For this review, use the dimensioned drawing (mm, ordinates from the lowest corner) and the shaded views. Coordinates: 2 decimals unless noted, no trailing zeros. Write each loop counter-clockwise with the first axis right and the second up, starting at its lowest first coordinate (ties: lowest second). Pieces come first, ordered by that corner, then holes. Notation, with made-up numbers: (42.5, 29.5) -> (57.5, 29.5) arc R20 cw to (57.5, 49.5) -> close; hole circle Ø9 at (9.5, 80). An arc over 180 degrees is marked (long way). Put each result on its own line as item: value. Start each with the question number.
Item 1: To check wall thickness, follow L1, parallel to Y at x = 68.5, z = 4; L2, parallel to X at y = 7, z = 1.1; L3, parallel to Y at x = 55, z = 0.9. State the ranges of each line that lie inside material, in increasing order.
Item 2: Consider section D-D on x = 30.5. Give the boundary of the cut face in (y, z).
Item 3: Consider section B-B on z = 3.05. Give the boundary of the cut face in (x, y).
Item 4: Consider section C-C on y = 29.5. Give the boundary of the cut face in (x, z), and give its area (3 significant figures).
Item 5: Consider section A-A on y = 8.5. Give the boundary of the cut face in (x, z), and give its area (3 significant figures).
Item 6: Insertion check: P1, Ø1, axis at x = 55, z = 2, coming from the +Y side; P2, Ø1.4, axis at y = 32, z = 2, coming from the -X side; P3, Ø1.4, axis at y = 2, z = 2.5, coming from the -X side. Each pin has a flat end and moves straight along its axis. Give the tip position at first contact, or say it passes through.
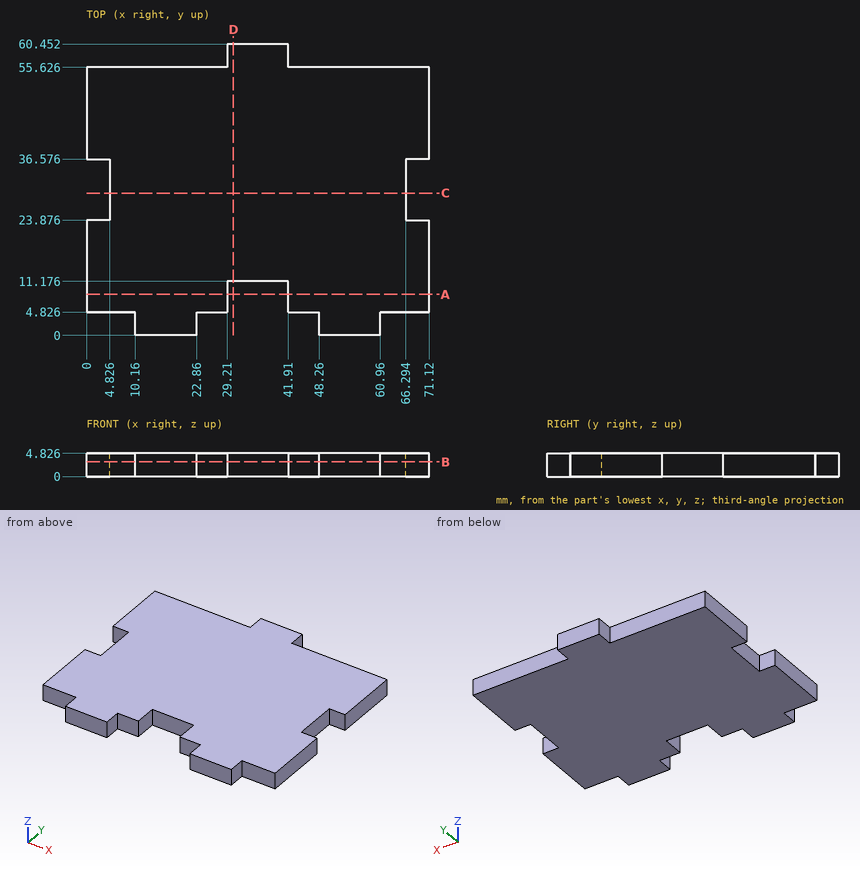
Return value:
1. L1: 4.83 to 23.88, 36.58 to 55.63
1. L2: 0 to 29.21, 41.91 to 71.12
1. L3: 0 to 55.63
2. outline: (11.18, 0) -> (60.45, 0) -> (60.45, 4.83) -> (11.18, 4.83) -> close
3. outline: (0, 4.83) -> (10.16, 4.83) -> (10.16, 0) -> (22.86, 0) -> (22.86, 4.83) -> (29.21, 4.83) -> (29.21, 11.18) -> (41.91, 11.18) -> (41.91, 4.83) -> (48.26, 4.83) -> (48.26, 0) -> (60.96, 0) -> (60.96, 4.83) -> (71.12, 4.83) -> (71.12, 23.88) -> (66.29, 23.88) -> (66.29, 36.58) -> (71.12, 36.58) -> (71.12, 55.63) -> (41.91, 55.63) -> (41.91, 60.45) -> (29.21, 60.45) -> (29.21, 55.63) -> (0, 55.63) -> (0, 36.58) -> (4.83, 36.58) -> (4.83, 23.88) -> (0, 23.88) -> close
4. outline: (4.83, 0) -> (66.29, 0) -> (66.29, 4.83) -> (4.83, 4.83) -> close
4. area: 297 mm^2
5. outline: (0, 0) -> (29.21, 0) -> (29.21, 4.83) -> (0, 4.83) -> close; (41.91, 0) -> (71.12, 0) -> (71.12, 4.83) -> (41.91, 4.83) -> close
5. area: 282 mm^2
6. P1: y = 55.63
6. P2: x = 4.83
6. P3: x = 10.16
